Input: part model. Units: mm. Frame: model coordinates. Coordinates: 2 decimals unless noted, no trailing zeros. Loops run counter-clockwise (first coordinate to the right, second up) from the corner with the lowest first, then second, coordinate; pieces in that order, holes last. Notation, with made-up numbers: (45, 60) -> (57, 60) arc R20 cw to (57, 91) -> close; hole circle Ø10 at (27.25, -5). An arc over 180 degrees is marked (long way). Put each result on its own line as item: value. Start each with the question number.
1) Material intervals for L1, parallel to Y at x = 34, z = 0.5, sorted ascending.
2) Cut plane B-B (z = 1.5). Return the cut outline in (x, y), plus the area to 3 significant figures.
3) Cut plane A-A (x = 16.5). Return the cut outline in (y, z), plus the area to 3 significant figures.
4) Pull-direction query (Z, two-part tool) for faces 1 (the flat face through (21, 38, 6.3)), 2 (the flat face through (21, 0, 3)), 3 (the flat face through (21, 38, 0)); classes: pulls with the +Z half, pulls with the -Z half, needs draft (parallel to the pull), parting line crosses it, or undercut.
Autodesk Fusion 360 part; units mm, degrees
box "BoxPrimitive1" add length 76.5 width 42 height 6.3 placed x (0, 1, 0) y (-1, 0, 0) z (0, 0, 1) at (42, 0, 0)
cylinder "CylinderPrimitive1" add diameter 1.5 height 20 placed x (1, 0, 0) y (0, 0, 1) z (0, -1, 0) at (39.3422, 0, 3.15)
cylinder "CylinderPrimitive2" add diameter 1.5 height 20 placed x (1, 0, 0) y (0, 0, 1) z (0, -1, 0) at (37.5, 0, 3.15)
Results found:
1. L1: y = 0 to 76.5
2. outline: (0, 0) -> (42, 0) -> (42, 76.5) -> (0, 76.5) -> close
2. area: 3,210 mm2
3. outline: (0, 0) -> (76.5, 0) -> (76.5, 6.3) -> (0, 6.3) -> close
3. area: 482 mm2
4. face 1: pulls with the +Z half
4. face 2: needs draft
4. face 3: pulls with the -Z half
